Check sheet for the modelled part. Datum: model origin and axes. Units: mm. Face numbers are marked on the shaded views. A direction names the side the tool comes from. Give positions to 0.01 mm unless a question says otherwise; leave off trailing zeros. Loops run counter-clockwise (first coordinate to the right, second up) from the corner with the lowest first, then second, coordinate; pieces in that order, holes last. Notation, with made-up numbers: M -24,0.5 L 4,0.5 A7 cw 4,4.5 Z; hole C 87,44 d5. An arc over 180 degrees is marked long. Use one line per item in the form item = value.
from build123d import *

# Parameters (mm, degrees)
SCHIZZO1_W                   = 50
SCHIZZO1_H                   = 50
ESTRUSIONE_ESTRUSIONE1_DEPTH = 50


with BuildPart() as part:
    # Schizzo1 → Estrusione-Estrusione1 (new body)
    with BuildSketch(Plane.XY):
        with Locations((25, 75)):
            Rectangle(SCHIZZO1_W, SCHIZZO1_H)
        with Locations((25, 25)):
            Rectangle(SCHIZZO1_W, SCHIZZO1_H)
        Polygon((50, 50), (50, 0), (100, 0), (100, 25), (100, 50), align=None)
        Polygon((50, 100), (50, 50), (100, 50), (100, 75), (100, 100), align=None)
        with Locations((125, 50)):
            Rectangle(SCHIZZO1_W, SCHIZZO1_H)
    extrude(amount=ESTRUSIONE_ESTRUSIONE1_DEPTH)


solid = part.part
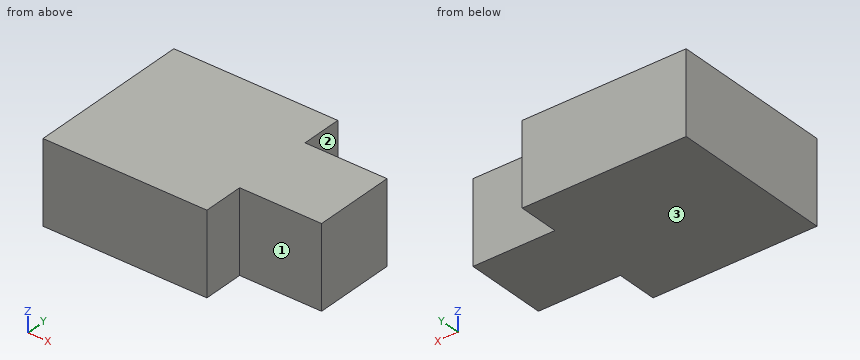
1) Section check B-B (y = 81). Record the cut outline in (x, z), then the cut area to 3 significant figures.
Evaluation:
outline = M 0,0 L 100,0 L 100,50 L 0,50 Z
area = 5,000 mm^2
2) Section check C-C (x = 111). Record the cut outline in (y, z), then the cut area to 3 significant figures.
Evaluation:
outline = M 25,0 L 75,0 L 75,50 L 25,50 Z
area = 2,500 mm^2
3) Scan lines: line 1 (X direction, y = 19, z = 4.5); line 2 (Y direction, x = 101.5, z = 27). Record each from-to range of solid material in increasing order.
Evaluation:
line_1 = 0 to 100
line_2 = 25 to 75
4) Set-up check for the marked faces 1, 2 and 3: record each of +Z, -Z, +X, -X, +Y, -Y from which the full face is reachable in a straight line by a thin tool's end or side.
Evaluation:
face_1 = +Z, -Z, +X, -Y
face_2 = +Z, -Z, +X, +Y
face_3 = -Z, +X, -X, +Y, -Y
5) Depth check by flat-ended pin: pin 1 Ø7.5 at (y, z) = (8, 13.5) entering from +X; pin 2 Ø2 at (x, z) = (117, 33) entering from +Y. Enter the tip coordinate at first touch or a pass-through.
Evaluation:
pin_1 = 100
pin_2 = 75
6) Section check A-A (z = 21.5). Record the cut outline in (x, y).
Evaluation:
outline = M 0,0 L 100,0 L 100,25 L 150,25 L 150,75 L 100,75 L 100,100 L 0,100 Z
